from build123d import *

# Parameters (mm, degrees)
SKETCH1_R          = 4.5
BASE_FLANGE1_DEPTH = 3


# Sheet-metal steps are written as plain solids
with BuildPart() as part:
    # Sketch1 → Base-Flange1 (new body)
    with BuildSketch(Plane(origin=(0, 0, 0), x_dir=(1, 0, 0), z_dir=(0, 1, 0))):
        Polygon((411.5, 275), (463.5, 275), (463.5, 180), (411.5, 180), (411.5, -275), (-411.5, -275), (-411.5, 275), align=None)
        with Locations(Location((-39, -212, 0), (0, 0, 90))):
            Circle(SKETCH1_R, mode=Mode.SUBTRACT)
        with Locations(Location((-39, -20, 0), (0, 0, 270))):
            Circle(SKETCH1_R, mode=Mode.SUBTRACT)
        with Locations(Location((40, -20, 0), (0, 0, 90))):
            Circle(SKETCH1_R, mode=Mode.SUBTRACT)
        with Locations(Location((40, -212, 0), (0, 0, 270))):
            Circle(SKETCH1_R, mode=Mode.SUBTRACT)
    extrude(amount=-BASE_FLANGE1_DEPTH)


solid = part.part
Verification items for the finished model (mm, model axes). Coordinates: 2 decimals unless noted, no trailing zeros. Order: outer loops, then holes, each group sorted by start corner. A loop starts at its lowest first (then second) coordinate and runs counter-clockwise, first axis right, second up. Notation, with made-up numbers: M -10,9.25 L 29,9.25 A34 cw 29,48.25 Z; hole C -18.5,35 d1. An arc over 180 degrees is marked long. One line per item, written item: value. Start each with the question number.
Item 1: Sectioned sample at A-A on y = -1.2. Record the cut outline in (x, z), then the cut area to 3 significant figures.
Item 2: Sectioned sample at B-B on z = 96. Record the cut outline in (x, y).
Item 3: Thickness scan on probe 1 along X at (y, z) = (-1.6, 20); probe 2 along Z at (x, y) = (-39.5, -2.7); probe 3 along X at (y, z) = (-0.5, 176.5). Record the ranges inside material, lowest first.
Item 4: Depth check by flat-ended pin: P1, Ø6, axis at x = 237, z = -15.5, coming from the +Y side; P2, Ø0.9, axis at x = 437, y = -1, coming from the +Z side; P3, Ø8, axis at x = 40, z = 20, coming from the +Y side; P4, Ø1.5, axis at y = -1, z = -48.5, coming from the +X side. Enter the tip coordinate at first touch or a pass-through.
Calculated:
1. outline: M -411.5,-275 L 463.5,-275 L 463.5,-180 L 411.5,-180 L 411.5,275 L -411.5,275 Z; hole C -39,20 d9; hole C -39,212 d9; hole C 40,20 d9; hole C 40,212 d9
1. area: 457,000 mm^2
2. outline: M -411.5,-3 L 411.5,-3 L 411.5,0 L -411.5,0 Z
3. probe 1: -411.5 to -43.5, -34.5 to 35.5, 44.5 to 411.5
3. probe 2: -275 to 15.53, 24.47 to 207.53, 216.47 to 275
3. probe 3: -411.5 to 411.5
4. P1: y = 0
4. P2: z = -180
4. P3: through
4. P4: x = 411.5
